Can you work these out from the model? Positions are in its coordinate system, mm. A direction names the side the tool comes from. Round coordinates to 2 decimals unless told otherwise and drop trailing zeros. Order: outer loops, then holes, each group sorted by start corner. A loop starts at its lowest first (then second) coordinate and runs counter-clockwise, first axis right, second up. Notation, with made-up numbers: (81, 30.5) -> (122, 30.5) arc R16 ccw to (122, 39.5) -> close; hole circle Ø2 at (-24.75, -34). An arc over 180 degrees is marked (long way). Use a Markdown table: item, result. Add a question column.
Q1. If we section it at D-D on y = 75: List the corners of the cut face in (x, z) for me, plus the area to 3 significant figures.
Q2. For faces 4 (the face through (-1, 0, 45)), 5 (the face through (-1, 0, -44)), 6 (the face through (1.5, -3.2, 0.1)), which set-ups out of +Z, -Z, +X, -X, +Y, -Y let a thin tool reach every point of the face, with its end or its side?
Q3. I'm going to push flat-ended pins straight in: pin 1 Ø4 at (y, z) = (14.5, -11.5) entering from +X; pin 2 Ø5 at (y, z) = (42.5, 11) entering from +X; pin 3 Ø4 at (y, z) = (33, -23.5) entering from -X. Where does each tip first touch, or does it pass through?
Q4. If we section it at A-A on z = 0: List the corners of the cut face in (x, y) for me (3 decimals), plus the area to 3 significant figures.
Q5. If we section it at C-C on z = -14: List the corners of the cut face in (x, y) for me (3 decimals).
Q6. If we section it at B-B on x = 0: List the corners of the cut face in (y, z) for me (3 decimals).
Q7. I need wall thicknesses on line 1 along X through (y, z) = (40, 0); line 2 along Z through (x, y) = (33, 34). Which ranges of each line are inside material? Lowest first, please. Write a range as [from, to].
Q8. We'd pull the mould along Z, two halves only. Please class faces 1 (the face through (1.467, -10.658, 0.469)), 2 (the face through (-1, 0, 7)), 3 (the face through (104.775, 2, 3)): +Z half, -Z half, draft (parallel to the pull), parting line (faces both ways), or undercut.
```python
from build123d import *

# Parameters (mm, degrees)
F2_R          = 10.668
F3_DEPTH      = 104.775
F3_DEPTH_BACK = 104.775
F0_R          = 57.15
F4_DEPTH      = 104.775
F5_R          = 3.2004
F6_DEPTH      = 209.551
F1_R          = 40.0304
F7_DEPTH      = 104.776


with BuildPart() as f3:
    # F2 (on Right) → F3 (new body, two sides)
    with BuildSketch(Plane.YZ) as f3_sk:
        Circle(F2_R)
    extrude(amount=F3_DEPTH)
    extrude(f3_sk.sketch, amount=-F3_DEPTH_BACK)

    # F0 (on Front) → F4 (join)
    with BuildSketch(Plane.XZ):
        Circle(F0_R)
    extrude(amount=-F4_DEPTH)

    # F5 (on face) → F6 (cut, through all)
    with BuildSketch(Plane.YZ.offset(104.775)):
        Circle(F5_R)
    extrude(amount=-F6_DEPTH, mode=Mode.SUBTRACT)

    # F1 (on Front) → F7 (cut, through all)
    with BuildSketch(Plane.XZ):
        Circle(F1_R)
    extrude(amount=-F7_DEPTH, mode=Mode.SUBTRACT)


solid = f3.part
```
Answer below:
| question | item | result |
|---|---|---|
| 1 | outline | circle Ø114.3 at (0, 0); hole circle Ø80.06 at (0, 0) |
| 1 | area | 5,230 mm² |
| 2 | face 4 | +Z, +X, -X, -Y |
| 2 | face 5 | -Z, +X, -X, -Y |
| 2 | face 6 | +X, -X |
| 3 | pin 1 | x = 56.35 |
| 3 | pin 2 | x = 56.51 |
| 3 | pin 3 | x = -52.95 |
| 4 | outline | (-104.775, -10.668) -> (104.775, -10.668) -> (104.775, -3.2) -> (-104.775, -3.2) -> close; (-104.775, 3.2) -> (-40.03, 3.2) -> (-40.03, 104.775) -> (-57.15, 104.775) -> (-57.15, 10.668) -> (-104.775, 10.668) -> close; (40.03, 3.2) -> (104.775, 3.2) -> (104.775, 10.668) -> (57.15, 10.668) -> (57.15, 104.775) -> (40.03, 104.775) -> close |
| 4 | area | 5,750 mm² |
| 5 | outline | (-55.409, 0) -> (-37.502, 0) -> (-37.502, 104.775) -> (-55.409, 104.775) -> close; (37.502, 0) -> (55.409, 0) -> (55.409, 104.775) -> (37.502, 104.775) -> close |
| 6 | outline | (0, -57.15) -> (104.775, -57.15) -> (104.775, -40.03) -> (0, -40.03) -> close; (0, -10.668) -> (0, -3.2) arc R3.2 cw to (0, 3.2) -> (0, 10.668) arc R10.668 ccw to start; (0, 40.03) -> (104.775, 40.03) -> (104.775, 57.15) -> (0, 57.15) -> close |
| 7 | line 1 | [-57.15, -40.03], [40.03, 57.15] |
| 7 | line 2 | [-46.66, -22.66], [22.66, 46.66] |
| 8 | face 1 | parting line |
| 8 | face 2 | undercut |
| 8 | face 3 | draft |
